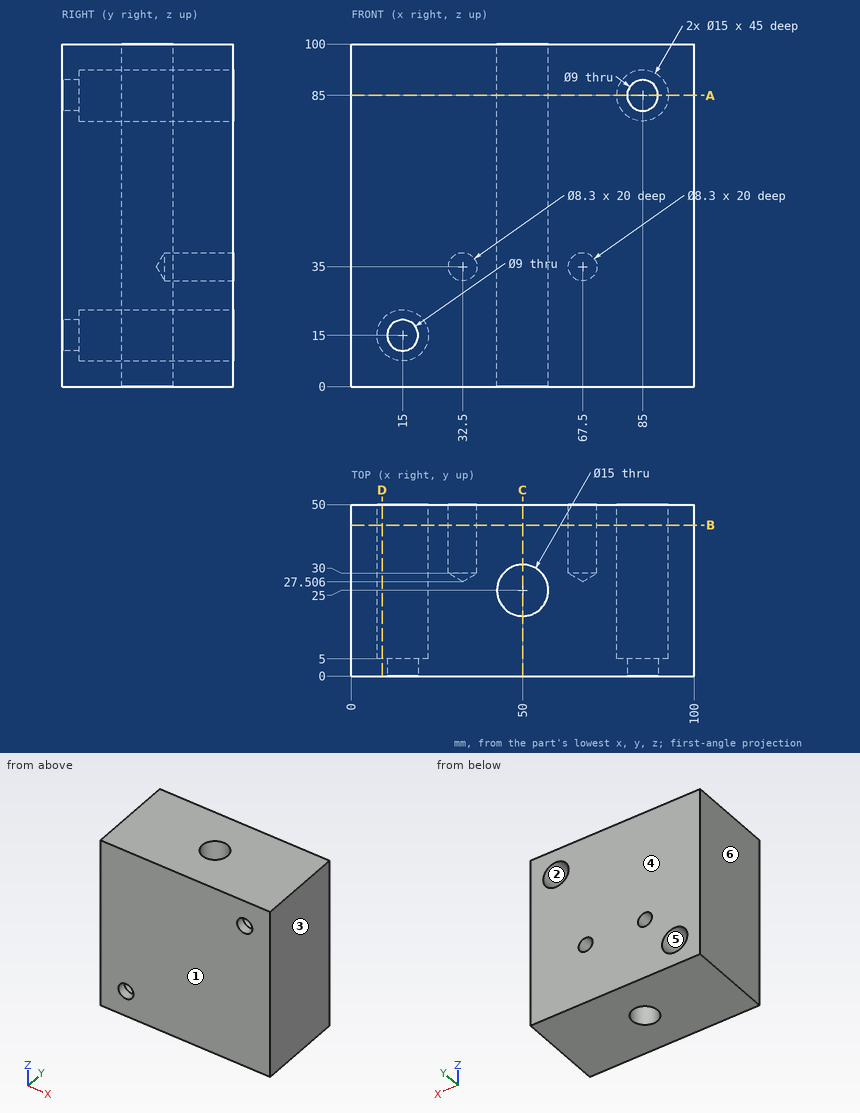
The drawing under review shows one solid part. Ordinate dimensions are in mm from its lowest x, y, z. A direction names the side the tool comes from. Give positions to 0.01 mm unless a question says otherwise; leave off trailing zeros. Loops run counter-clockwise (first coordinate to the right, second up) from the corner with the lowest first, then second, coordinate; pieces in that order, holes last. Notation, with made-up numbers: M 4,83.5 L 40,83.5 A25 ccw 40,115.5 Z; hole C 43,39 d1. An arc over 180 degrees is marked long. Return JSON: item names as keys, results as strings. Group by question number.
Item 1: Tool access review of the marked faces 1 and 2: name each direction out of +Z, -Z, +X, -X, +Y, -Y from which nothing blocks a thin tool from reaching the whole face with its end or side.
Item 2: For probe 1 along X at (y, z) = (35, 85); probe 2 along Z at (x, y) = (32, 42); probe 3 along Z at (x, y) = (85, 3), list the stretches that pass through material, from the lowest coordinate up.
Item 3: We need section B-B (y = 44). Give the boundary of the cut face in (x, z), and give its area (3 significant figures).
Item 4: Insertion check: pin 1 Ø13.5 at (x, y) = (50, 25) entering from +Z; pin 2 Ø4.5 at (x, z) = (86, 88) entering from +Y. Each pin has a flat end and moves straight along its axis. Give the tip position at first contact, or say it passes through.
Item 5: We need section D-D (x = 9). Give the boundary of the cut face in (y, z).
Item 6: We need section C-C (x = 50). Give the boundary of the cut face in (y, z).
Item 7: Mouldability with a two-part tool opening along X and no side actions: class the marked faces 3, 4, 5 and 6 as released by +X, released by -X, zero draft, split by the parting line, or undercut.
Item 8: We need section A-A (z = 85). Give the boundary of the cut face in (x, y), and give its area (3 significant figures).
Output:
{
 "1": {"face 1": "+Z, -Z, +X, -X, -Y", "face 2": "+Y"},
 "2": {"probe 1": "x = 0 to 77.5, 92.5 to 100", "probe 2": "z = 0 to 30.88, 39.12 to 100", "probe 3": "z = 0 to 80.5, 89.5 to 100"},
 "3": {"outline": "M 0,0 L 100,0 L 100,100 L 0,100 Z; hole C 15,15 d15; hole C 32.5,35 d8.3; hole C 67.5,35 d8.3; hole C 85,85 d15", "area": "9,540 mm^2"},
 "4": {"pin 1": "passes through", "pin 2": "stops at y = 5"},
 "5": {"outline": "M 0,0 L 50,0 L 50,10.5 L 5,10.5 L 5,19.5 L 50,19.5 L 50,100 L 0,100 Z"},
 "6": {"outline": "M 0,0 L 17.5,0 L 17.5,100 L 0,100 Z; M 32.5,0 L 50,0 L 50,100 L 32.5,100 Z"},
 "7": {"face 3": "released by +X", "face 4": "zero draft", "face 5": "undercut", "face 6": "released by -X"},
 "8": {"outline": "M 0,0 L 80.5,0 L 80.5,5 L 77.5,5 L 77.5,50 L 0,50 Z; M 89.5,0 L 100,0 L 100,50 L 92.5,50 L 92.5,5 L 89.5,5 Z; hole C 50,25 d15", "area": "4,100 mm^2"}
}
